from build123d import *

# Parameters (mm, degrees)
ESQUISSE1_R        = 1.9
ESQUISSE1_R_2      = 4.5
ESQUISSE1_W        = 8
ESQUISSE1_H        = 5
BOSS_EXTRU_1_DEPTH = 5


with BuildPart() as part:
    # Esquisse1 → Boss.-Extru.1 (new body)
    with BuildSketch(Plane.XY):
        with BuildLine():
            Line((-22.984184861, -5.970148314), (-31.145801552, -8.941620925))
            ThreePointArc((-31.145801552, -8.941620925), (-34.899958966, -15.635885981), (-29, -20.544792857))
            Line((-29, -20.544792857), (26, -20.544792857))
            ThreePointArc((26, -20.544792857), (34.902651948, -10.224645785), (23.388264466, -2.932079143))
            ThreePointArc((23.388264466, -2.932079143), (20.213182454, -3.358665896), (17.066134535, -2.7593234))
            Line((17.066134535, -2.7593234), (6.175413191, 1.204575468))
            ThreePointArc((6.175413191, 1.204575468), (1.404093414, 4.865736977), (-0.404386386, 10.601501853))
            Line((-0.404386386, 10.601501853), (-0.404386386, 12.54541747))
            ThreePointArc((-0.404386386, 12.54541747), (-8.404386386, 20.54541747), (-16.404387146, 12.54541747))
            Line((-16.404387146, 12.54541747), (-16.404387146, 3.426777584))
            ThreePointArc((-16.404387146, 3.426777584), (-18.212866443, -2.308986408), (-22.984184861, -5.970148314))
        make_face()
        with Locations((-8.404386386, 12.54541747)):
            Circle(ESQUISSE1_R, mode=Mode.SUBTRACT)
        with Locations((-29, -14.544792857)):
            Circle(ESQUISSE1_R, mode=Mode.SUBTRACT)
        with Locations((26, -11.544792857)):
            Circle(ESQUISSE1_R_2, mode=Mode.SUBTRACT)
        with Locations((4.999995852, -14.564792857)):
            Rectangle(ESQUISSE1_W, ESQUISSE1_H, mode=Mode.SUBTRACT)
        Polygon((-17.000004148, -12.064792857), (-17.013857883, -17.064792857), (-9.000004148, -17.064792857), (-9.000004148, -12.064792857), align=None, mode=Mode.SUBTRACT)
    extrude(amount=BOSS_EXTRU_1_DEPTH)


solid = part.part
The model under review builds one solid part; all positions refer to its coordinate system, in mm. A direction names the side the tool comes from. Round coordinates to 2 decimals unless told otherwise and drop trailing zeros. Loops run counter-clockwise (first coordinate to the right, second up) from the corner with the lowest first, then second, coordinate; pieces in that order, holes last. Notation, with made-up numbers: (22.5, 78) -> (60.5, 78) arc R25 ccw to (60.5, 96) -> close; hole circle Ø1 at (85, 59). An arc over 180 degrees is marked (long way). Write item = value, one per line. Start each with the question number.
Item 1: Insertion check: pin 1 (1.5 mm diameter, centred on x = -0.5, z = 1, fed in from +Y); pin 2 (0.6 mm diameter, centred on y = 11.5, z = 1.5, fed in from +X); pin 3 (2.5 mm diameter, centred on x = -11, z = 3, fed in from +Y). Each pin has a flat end and moves straight along its axis. Give the tip position at first contact, or say it passes through.
Item 2: Take a section at A-A on x = 4. Give the boundary of the cut face in (y, z), plus the area to 3 significant figures.
Item 3: Mouldability with a two-part tool opening along X and no side actions: class faces 1 (the cylindrical face through (1.45, 4.8, 2.46)), 2 (the cylindrical face through (-34.92, -15.52, 2.46)), 3 (the cylindrical face through (-27.245, -15.273, 2.465)) as released by +X, released by -X, zero draft, split by the parting line, or undercut.
Item 4: Take a section at C-C on y = -10.5. Give the boundary of the cut face in (x, z).
Item 5: For faces 4 (the flat face through (-9, -15, 2)), 5 (the flat face through (-16.404, 8, 2)), 6 (the flat face through (-0.404, 12, 2)), list the 3-axis set-ups (+Z, -Z, +X, -X, +Y, -Y) from which the entire face can be reached by the end or side of a thin tool; tool diameter is ignored.
Item 6: Take a section at D-D on y = 8. Give the boundary of the cut face in (x, z), plus the area to 3 significant figures.
Item 7: Take a section at B-B on z = 1.6. Give the boundary of the cut face in (x, y).
Item 8: To check wall thickness, follow L1, parallel to X at y = -17, z = 1.9; L2, parallel to Y at x = -10, z = 3.7; L3, parallel to Y at x = 23, z = 0.65. State the ranges of each line that lie inside material, in increasing order.
Result:
q1.pin_1 = 16.13
q1.pin_2 = -0.4
q1.pin_3 = 20.43
q2.outline = (-20.54, 0) -> (-17.06, 0) -> (-17.06, 5) -> (-20.54, 5) -> close; (-12.06, 0) -> (2.31, 0) -> (2.31, 5) -> (-12.06, 5) -> close
q2.area = 89.3 mm²
q3.face_1 = released by +X
q3.face_2 = released by -X
q3.face_3 = undercut
q4.outline = (-33.43, 0) -> (21.62, 0) -> (21.62, 5) -> (-33.43, 5) -> close; (30.38, 0) -> (34.94, 0) -> (34.94, 5) -> (30.38, 5) -> close
q5.face_4 = +Z, -Z
q5.face_5 = +Z, -Z, -X, +Y
q5.face_6 = +Z, -Z, +X, +Y
q6.outline = (-16.4, 0) -> (-0.06, 0) -> (-0.06, 5) -> (-16.4, 5) -> close
q6.area = 81.7 mm²
q7.outline = (-31.15, -8.94) arc R6 ccw to (-29, -20.54) -> (26, -20.54) arc R9 ccw (long way) to (23.39, -2.93) arc R10 cw to (17.07, -2.76) -> (6.18, 1.2) arc R10 cw to (-0.4, 10.6) -> (-0.4, 12.55) arc R8 ccw to (-16.4, 12.55) -> (-16.4, 3.43) arc R10 cw to (-22.98, -5.97) -> close; hole circle Ø3.8 at (-29, -14.54); hole (-17.01, -17.06) -> (-9, -17.06) -> (-9, -12.06) -> (-17, -12.06) -> close; hole circle Ø3.8 at (-8.4, 12.55); hole (1, -17.06) -> (9, -17.06) -> (9, -12.06) -> (1, -12.06) -> close; hole circle Ø9 at (26, -11.54)
q8.L1 = -34.47 to -17.01, -9 to 1, 9 to 33.16
q8.L2 = -20.54 to -17.06, -12.06 to 11.51, 13.58 to 20.38
q8.L3 = -20.54 to -14.9, -8.19 to -3.04
